Could you check a few things on this model? Use its own coordinates, in mm. Face numbers are marked on the shaded views. A direction names the side the tool comes from. Round coordinates to 2 decimals unless told otherwise and drop trailing zeros. Loops run counter-clockwise (first coordinate to the right, second up) from the corner with the lowest first, then second, coordinate; pieces in that order, holes last. Notation, with made-up numbers: (9.25, 9) -> (47.25, 9) arc R7 ccw to (47.25, 16) -> close; hole circle Ø4 at (79, 1.5). An arc over 180 degrees is marked (long way). One line per item, written item: value.
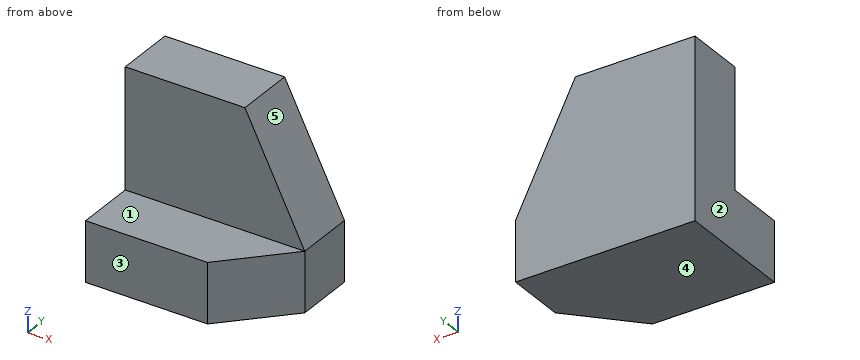
```python
from build123d import *

# Parameters (mm, degrees)
F2_DEPTH = 25.4
F4_DEPTH = 25.4
F5_W     = 12.7
F5_H     = 25.4
F6_DEPTH = 38.1
F8_DEPTH = 25.4


with BuildPart() as f2:
    # F1 (on face) → F2 (new body)
    with BuildSketch(Plane.XZ):
        Polygon((38.1, 38.1), (0, 38.1), (0, 0), (38.1, 0), (38.1, 13.111571), align=None)
    extrude(amount=F2_DEPTH)

    # F3 (on face) → F4 (cut)
    with BuildSketch(Plane.XZ.offset(25.4)):
        Polygon((25.4, 38.1), (38.1, 12.7), (38.1, 38.1), align=None)
    extrude(amount=-F4_DEPTH, mode=Mode.SUBTRACT)

    # F5 (on face) → F6 (cut)
    with BuildSketch(Plane(origin=(0, 0, 0), x_dir=(0, -1, 0), z_dir=(-1, 0, 0))):
        with Locations((19.05, 25.4)):
            Rectangle(F5_W, F5_H)
    extrude(amount=-F6_DEPTH, mode=Mode.SUBTRACT)

    # F7 (on face) → F8 (cut)
    with BuildSketch(Plane.XY.offset(12.7)):
        Polygon((38.1, -25.4), (38.1, -12.7), (25.894709, -25.4), align=None)
    extrude(amount=-F8_DEPTH, mode=Mode.SUBTRACT)


solid = f2.part
```
Item 1: If we mould it in two halves opening along Z, with no side actions, what happens to the marked faces 3, 4 and 5? For each: released by +Z, released by -Z, zero draft, split by the parting line, or undercut.
Output:
face 3: zero draft
face 4: released by -Z
face 5: released by +Z
Item 2: If we section it at D-D on z = 19: List the corners of the cut face in (x, y) for me, plus the area to 3 significant figures.
Output:
outline: (0, -12.7) -> (34.95, -12.7) -> (34.95, 0) -> (0, 0) -> close
area: 444 mm²
Item 3: If we section it at C-C on y = -7: List the corners of the cut face in (x, z) for me, plus the area to 3 significant figures.
Output:
outline: (0, 0) -> (38.1, 0) -> (38.1, 12.7) -> (25.4, 38.1) -> (0, 38.1) -> close
area: 1,290 mm²
Item 4: If we section it at A-A on x = 10.5: List the corners of the cut face in (y, z) for me, plus the area to 3 significant figures.
Output:
outline: (-25.4, 0) -> (0, 0) -> (0, 38.1) -> (-12.7, 38.1) -> (-12.7, 12.7) -> (-25.4, 12.7) -> close
area: 645 mm²
Item 5: Will these pins go through, and if not, where does the flat tip stop? pin 1 Ø7.5 at (x, z) = (17, 30.5) entering from -Y; pin 2 Ø6.5 at (x, y) = (19, -19) entering from +Z.
Output:
pin 1: stops at y = -12.7
pin 2: stops at z = 12.7
Item 6: I need wall thicknesses on line 1 (Z direction, x = 33.5, y = -15.25); line 2 (Y direction, x = 12, z = 36); line 3 (X direction, y = -3.25, z = 18). Which ranges of each line are inside material? Lowest first, please. Write a range as from..to.
Output:
line 1: z = 0..12.7
line 2: y = -12.7..0
line 3: x = 0..35.45
Item 7: For the marked faces 1 and 2, which set-ups out of +Z, -Z, +X, -X, +Y, -Y let a thin tool reach every point of the face, with its end or its side?
Output:
face 1: +Z, +X, -X, -Y
face 2: +Z, -Z, -X, +Y, -Y
Item 8: If we section it at B-B on z = 3: List the corners of the cut face in (x, y) for me, plus the area to 3 significant figures.
Output:
outline: (0, -25.4) -> (25.89, -25.4) -> (38.1, -12.7) -> (38.1, 0) -> (0, 0) -> close
area: 890 mm²
